For this review, use the dimensioned drawing (mm, ordinates from the lowest corner) and the shaded views. A direction names the side the tool comes from. Round coordinates to 2 decimals unless told otherwise and drop trailing zeros. Write each loop counter-clockwise with the first axis right and the second up, starting at its lowest first coordinate (ties: lowest second). Pieces come first, ordered by that corner, then holes.
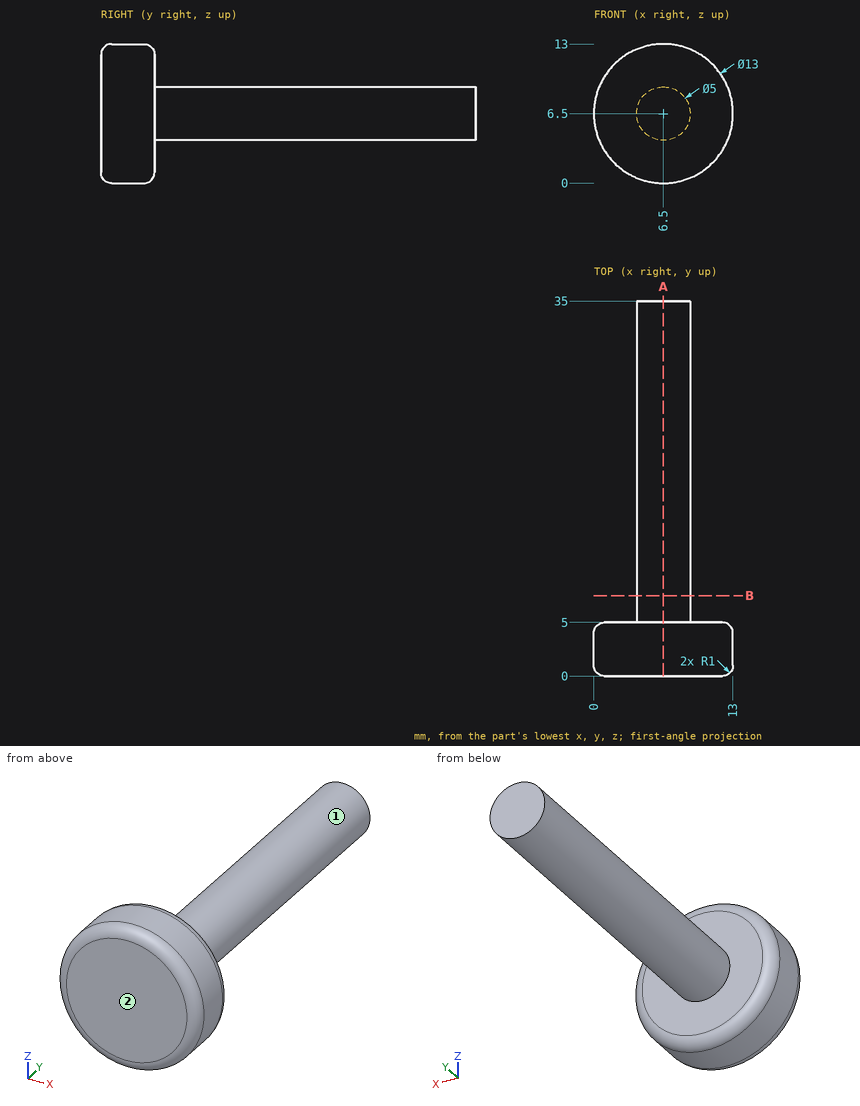
1) For the marked faces 1 and 2, list the 3-axis set-ups (+Z, -Z, +X, -X, +Y, -Y) from which the entire face can be reached by the end or side of a thin tool; tool diameter is ignored.
2) For P1, Ø5, axis at y = 16, z = 9, coming from the +X side; P2, Ø5, axis at x = 2.5, y = 27.5, coming from the +Z side; P3, Ø4, axis at x = 9.5, y = 17.5, coming from the -Z side, all flat-tipped, find the tip position at first contact; note any pin that passes through.
3) Add section A-A on x = 6.5. State the section outline as (y, z) points, and give its area (3 significant figures).
4) For line 1 along Y through (x, z) = (2.25, 7); line 2 along Z through (x, y) = (7.75, 24.5); line 3 along Z through (x, y) = (5.5, 8.5), list the stretches that pass through material, from the lowest coordinate up.
5) Add section B-B on y = 7.5. State the section outline as (x, z) points.
Computed:
1. face 1: +Y
1. face 2: +Z, -Z, +X, -X, -Y
2. P1: stops at x = 9
2. P2: stops at z = 8.5
2. P3: stops at z = 4.21
3. outline: (0, 1) arc R1 ccw to (1, 0) - (4, 0) arc R1 ccw to (5, 1) - (5, 4) - (35, 4) - (35, 9) - (5, 9) - (5, 12) arc R1 ccw to (4, 13) - (1, 13) arc R1 ccw to (0, 12) - close
3. area: 214 mm2
4. line 1: y = 0 to 5
4. line 2: z = 4.33 to 8.67
4. line 3: z = 4.21 to 8.79
5. outline: circle Ø5 at (6.5, 6.5)
